Geometry: final body of the model. Coordinates: model frame, mm. Give positions to 0.01 mm unless a question says otherwise; leave off trailing zeros. Loops run counter-clockwise (first coordinate to the right, second up) from the corner with the lowest first, then second, coordinate; pieces in that order, holes last. Notation, with made-up numbers: (-22.5, 11.5) - (29.5, 11.5) arc R11 cw to (29.5, 30.5) - close; hole circle Ø4 at (56, 18.25). An arc over 180 degrees is marked (long way). Answer in a Markdown table with one row per item.
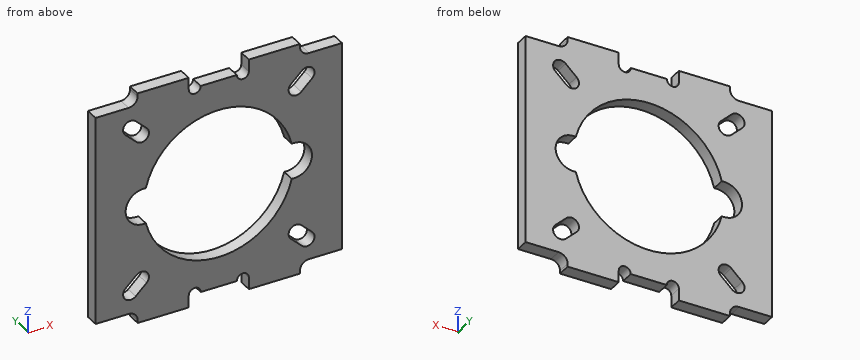
from build123d import *

# Parameters (mm, degrees)
SKETCH1_W            = 41
SKETCH1_H            = 39
BOSS_EXTRUDE1_DEPTH  = 2.2
SKETCH2_R            = 12.5
CUT_EXTRUDE1_DEPTH   = 29.378512998
SKETCH3_R            = 3
CUT_EXTRUDE2_DEPTH   = 29.378512998
SKETCH4_W            = 7
SKETCH4_H            = 2
CUT_EXTRUDE3_DEPTH   = 29.378512998
FILLET1_R            = 1.5
FILLET1_OF_MIRROR1_R = 1.5
MIRROR3_DEPTH        = 2.2


# Read off the part's stored shape, not the designer's step: Mirror3
with BuildPart() as part:
    # Sketch1 → Boss-Extrude1 (new body)
    with BuildSketch(Plane(origin=(0, 0, 0), x_dir=(1, 0, 0), z_dir=(0, 1, 0))):
        Rectangle(SKETCH1_W, SKETCH1_H)
    extrude(amount=BOSS_EXTRUDE1_DEPTH)

    # Sketch2 → Cut-Extrude1 (cut, through all)
    with BuildSketch(Plane(origin=(0, 0, 0), x_dir=(1, 0, 0), z_dir=(0, 1, 0))):
        with Locations(Location((0, 0, 0), (0, 0, 270))):
            Circle(SKETCH2_R)
    extrude(amount=CUT_EXTRUDE1_DEPTH, mode=Mode.SUBTRACT)

    # Sketch3 → Cut-Extrude2 (cut, through all)
    with BuildSketch(Plane(origin=(0, 0, 0), x_dir=(1, 0, 0), z_dir=(0, 1, 0))):
        with Locations((12.5, 0)):
            Circle(SKETCH3_R)
        with Locations((-12.5, 0)):
            Circle(SKETCH3_R)
        with BuildLine():
            Line((11.999388387, 13.139241924), (13.810783542, 14.862276339))
            ThreePointArc((13.810783542, 14.862276339), (15.577998326, 14.818095969), (15.533817957, 13.050881184))
            Line((15.533817957, 13.050881184), (13.722422802, 11.327846769))
            ThreePointArc((13.722422802, 11.327846769), (11.955208018, 11.372027139), (11.999388387, 13.139241924))
        make_face()
        with BuildLine():
            Line((11.999388387, -13.139241924), (13.810783542, -14.862276339))
            ThreePointArc((13.810783542, -14.862276339), (15.577998326, -14.818095969), (15.533817957, -13.050881184))
            Line((15.533817957, -13.050881184), (13.722422802, -11.327846769))
            ThreePointArc((13.722422802, -11.327846769), (11.955208018, -11.372027139), (11.999388387, -13.139241924))
        make_face()
        with BuildLine():
            Line((-11.999388387, -13.139241924), (-13.810783542, -14.862276339))
            ThreePointArc((-13.810783542, -14.862276339), (-15.577998326, -14.818095969), (-15.533817957, -13.050881184))
            Line((-15.533817957, -13.050881184), (-13.722422802, -11.327846769))
            ThreePointArc((-13.722422802, -11.327846769), (-11.955208018, -11.372027139), (-11.999388387, -13.139241924))
        make_face()
        with BuildLine():
            Line((-11.999388387, 13.139241924), (-13.810783542, 14.862276339))
            ThreePointArc((-13.810783542, 14.862276339), (-15.577998326, 14.818095969), (-15.533817957, 13.050881184))
            Line((-15.533817957, 13.050881184), (-13.722422802, 11.327846769))
            ThreePointArc((-13.722422802, 11.327846769), (-11.955208018, 11.372027139), (-11.999388387, 13.139241924))
        make_face()
    extrude(amount=CUT_EXTRUDE2_DEPTH, mode=Mode.SUBTRACT)

    # Sketch4 → Cut-Extrude3 (cut, through all)
    with BuildSketch(Plane(origin=(0, 0, 0), x_dir=(1, 0, 0), z_dir=(0, 1, 0))):
        with Locations((17, 18.5)):
            Rectangle(SKETCH4_W, SKETCH4_H)
        with BuildLine():
            Line((0, 19.5), (5, 19.5))
            Line((5, 19.5), (5, 17.5))
            ThreePointArc((5, 17.5), (4, 16.5), (3, 17.5))
            Line((3, 17.5), (0, 17.5))
            Line((0, 17.5), (0, 19.5))
        make_face()
    cut_extrude3 = extrude(amount=CUT_EXTRUDE3_DEPTH, mode=Mode.SUBTRACT)

    # Fillet1
    fillet1_edges = [part.edges().sort_by_distance(p)[0] for p in [
        (13.5, 1.1, -17.5),
    ]]
    fillet(fillet1_edges, radius=FILLET1_R)

    # Mirror1: Cut-Extrude3 across plane
    add(cut_extrude3.mirror(Plane(origin=(0, 0, 0), x_dir=(0, 0, 1), z_dir=(1, 0, 0))), mode=Mode.SUBTRACT)

    # Fillet1 of Mirror1
    fillet1_of_mirror1_edges = [part.edges().sort_by_distance(p)[0] for p in [
        (-13.5, 1.1, -17.5),
    ]]
    fillet(fillet1_of_mirror1_edges, radius=FILLET1_OF_MIRROR1_R)

    # Mirror3 outline → Mirror3 (cut)
    with BuildSketch(Plane(origin=(0, 0, 0), x_dir=(1, 0, 0), z_dir=(0, 1, 0))):
        with BuildLine():
            Line((-5, -19.5), (5, -19.5))
            Line((5, -19.5), (5, -17.5))
            ThreePointArc((5, -17.5), (4, -16.5), (3, -17.5))
            Line((3, -17.5), (-3, -17.5))
            ThreePointArc((-3, -17.5), (-4, -16.5), (-5, -17.5))
            Line((-5, -17.5), (-5, -19.5))
        make_face()
        with BuildLine():
            Line((13.5, -19), (13.5, -19.5))
            Line((13.5, -19.5), (20.5, -19.5))
            Line((20.5, -19.5), (20.5, -17.5))
            Line((20.5, -17.5), (15, -17.5))
            ThreePointArc((15, -17.5), (13.939339828, -17.939339828), (13.5, -19))
        make_face()
        with BuildLine():
            Line((-20.5, -19.5), (-13.5, -19.5))
            Line((-13.5, -19.5), (-13.5, -19))
            ThreePointArc((-13.5, -19), (-13.939339828, -17.939339828), (-15, -17.5))
            Line((-15, -17.5), (-20.5, -17.5))
            Line((-20.5, -17.5), (-20.5, -19.5))
        make_face()
    extrude(amount=MIRROR3_DEPTH, mode=Mode.SUBTRACT)


solid = part.part
Q1. Cut plane A-A (z = 0). Output: boundary loops of the cut face in (x, y).
Check values:
| item | result |
|---|---|
| outline | (-20.5, 0) - (-15.5, 0) - (-15.5, 2.2) - (-20.5, 2.2) - close; (15.5, 0) - (20.5, 0) - (20.5, 2.2) - (15.5, 2.2) - close |
Q2. Material intervals for line 1 along Z through (x, y) = (0, 2.05); line 2 along X through (y, z) = (0.8, 0); line 3 along Z through (x, y) = (-12.5, 0.7), sorted ascending.
Check values:
| item | result |
|---|---|
| line 1 | -17.5 to -12.5, 12.5 to 17.5 |
| line 2 | -20.5 to -15.5, 15.5 to 20.5 |
| line 3 | -19.5 to -13.62, -11.04 to -3, 3 to 11.04, 13.62 to 19.5 |
Q3. Cut plane C-C (y = 0.65). Give the number of separate pieces and of enclosed holes in the cut face, and give its area (3 significant figures).
Check values:
| item | result |
|---|---|
| separate pieces | 1 |
| enclosed holes | 5 |
| area | 933 mm² |
Q4. First-contact query: pin 1 (1 mm diameter, centred on y = 1, z = 18.5, fed in from -X); pin 2 (0.6 mm diameter, centred on y = 1, z = 19.5, fed in from -X); pin 3 (1.1 mm diameter, centred on x = 0, y = 0.5, fed in from +Z). Flat tips, straight axial feed; report the tip coordinate or a pass-through.
Check values:
| item | result |
|---|---|
| pin 1 | x = -13.88 |
| pin 2 | x = -13.5 |
| pin 3 | z = 17.5 |
Q5. Cut plane B-B (x = -3.5). Output: boundary loops of the cut face in (y, z), and give its area (3 significant figures).
Check values:
| item | result |
|---|---|
| outline | (0, -16.63) - (2.2, -16.63) - (2.2, -12) - (0, -12) - close; (0, 12) - (2.2, 12) - (2.2, 16.63) - (0, 16.63) - close |
| area | 20.4 mm² |
